Could you check a few things on this model? Use its own coordinates, in mm. Coordinates: 2 decimals unless noted, no trailing zeros. Order: outer loops, then holes, each group sorted by start corner. A loop starts at its lowest first (then second) coordinate and runs counter-clockwise, first axis right, second up. Notation, with made-up numbers: (52, 29) -> (91, 29) arc R34 cw to (91, 61) -> close; hole circle Ø7 at (3.5, -34.5). An arc over 180 degrees is marked (long way). Use a Markdown table: item, result. Add a question column.
1) If I drill on L1, parallel to X at y = 1.2, z = -79; L2, parallel to X at y = 3.2, z = -81, over which ranges is the centre line in solid material (lowest first)? Write a range as [from, to].
2) Thinking about a two-plate mould opening in X: for faces 1 (the flat face through (83, 0, -67)), 2 (the cylindrical face through (1.43, 2.54, -130.25)), 3 (the cylindrical face through (166.25, 2.54, -130.32)), 4 (the cylindrical face through (128.384, 2.535, -78.292)), which applies, +X half, -X half, draft (parallel to the pull), parting line (faces both ways), or undercut?
3) If we section it at A-A (z = -79.25): Write out the boundary of the cut face in (x, y) (3 decimals).
```python
from build123d import *

# Parameters (mm, degrees)
SKETCH_1_W          = 167.75
SKETCH_1_H          = 131.75
EXTRUDE_1_DEPTH     = 5
FILLET_1_R          = 5
FILLET_2_R          = 5
FILLET_3_R          = 5
FILLET_4_R          = 5
SKETCH_2_R          = 2.5
CUT_EXTRUDE_1_DEPTH = 10


with BuildPart() as part:
    # Эскиз1 → Бобышка-Вытянуть1 (new body)
    with BuildSketch(Plane(origin=(0, 0, 0), x_dir=(1, 0, 0), z_dir=(0, 1, 0))):
        with Locations((83.875, 65.875)):
            Rectangle(SKETCH_1_W, SKETCH_1_H)
    extrude(amount=EXTRUDE_1_DEPTH)

    # Скругление1
    fillet_1_edges = [part.edges().sort_by_distance(p)[0] for p in [
        (0, 2.5, 0),
    ]]
    fillet(fillet_1_edges, radius=FILLET_1_R)

    # Скругление2
    fillet_2_edges = [part.edges().sort_by_distance(p)[0] for p in [
        (0, 2.5, -131.75),
    ]]
    fillet(fillet_2_edges, radius=FILLET_2_R)

    # Скругление3
    fillet_3_edges = [part.edges().sort_by_distance(p)[0] for p in [
        (167.75, 2.5, -131.75),
    ]]
    fillet(fillet_3_edges, radius=FILLET_3_R)

    # Скругление4
    fillet_4_edges = [part.edges().sort_by_distance(p)[0] for p in [
        (167.75, 2.5, 0),
    ]]
    fillet(fillet_4_edges, radius=FILLET_4_R)

    # Эскиз2 → Вырез-Вытянуть1 (cut)
    with BuildSketch(Plane(origin=(0, 5, 0), x_dir=(1, 0, 0), z_dir=(0, 1, 0))):
        with Locations((126.075, 79.25)):
            Circle(SKETCH_2_R)
        with Locations((126.075, 52.5)):
            Circle(SKETCH_2_R)
        with Locations((41.675, 79.25)):
            Circle(SKETCH_2_R)
        with Locations((41.675, 52.5)):
            Circle(SKETCH_2_R)
    extrude(amount=-CUT_EXTRUDE_1_DEPTH, mode=Mode.SUBTRACT)


solid = part.part
```
Answer sheet:
| question | item | result |
|---|---|---|
| 1 | L1 | [0, 39.19], [44.16, 123.59], [128.56, 167.75] |
| 1 | L2 | [0, 39.89], [43.46, 124.29], [127.86, 167.75] |
| 2 | face 1 | draft |
| 2 | face 2 | -X half |
| 2 | face 3 | +X half |
| 2 | face 4 | undercut |
| 3 | outline | (0, 0) -> (39.175, 0) -> (39.175, 5) -> (0, 5) -> close; (44.175, 0) -> (123.575, 0) -> (123.575, 5) -> (44.175, 5) -> close; (128.575, 0) -> (167.75, 0) -> (167.75, 5) -> (128.575, 5) -> close |
